Build history of the part. All positions in model axes, mm. Face numbers are marked on the shaded views. Give positions to 0.01 mm unless a question says otherwise; leave off trailing zeros. Order: outer loops, then holes, each group sorted by start corner. A loop starts at its lowest first (then second) coordinate and runs counter-clockwise, first axis right, second up. Notation, with made-up numbers: (-4.5, 31.25) - (38.5, 31.25) arc R28 cw to (38.5, 64.25) - close; hole circle Ø1 at (59.5, 27). An arc over 180 degrees is marked (long way). Answer in a Markdown table with one row per item.
Autodesk Inventor part; units mm, degrees
ref_plane "YZ Plane" through (0, 0, 0) normal (1, 0, 0) x (0, 1, 0)
ref_plane "XZ Plane" through (0, 0, 0) normal (0, 1, 0) x (-1, 0, 0)
ref_plane "XY Plane" through (0, 0, 0) normal (0, 0, 1) x (1, 0, 0)
sketch "Sketch1" plane through (0, 0, 0) normal (0, 0, 1) x (1, 0, 0)
  circle A0 centre (0, 0) radius 15
  dimension "d0" = 30
extrude "Extrusion1" add sketch "Sketch1" along normal blind 40
sketch "Sketch2" plane through (0, 0, 40) normal (0, 0, 1) x (1, 0, 0)
  circle A0 centre (0, 0) radius 4
  dimension "d3" = 8
extrude "Extrusion2" cut sketch "Sketch2" against normal blind 40
sketch "Sketch3" plane through (0, 0, 40) normal (0, 0, 1) x (1, 0, 0)
  circle A0 centre (0, 0) radius 4
  circle A1 centre (0, 0) radius 15
  line L0 (0, 15) -> (1, 15)
  line L1 (0, 15) -> (-1, 15)
  line L2 (-0.0081, 4) -> (0.9843, 3.877)
  line L3 (-0.0081, 4) -> (-1, 3.873)
  line L4 (-1, 3.873) -> (-1, 15)
  line L5 (0.9843, 3.877) -> (1, 15)
  dimension "d8" = 1
  dimension "d9" = 1
  dimension "d10" = 1
  dimension "d11" = 1
extrude "Extrusion3" cut sketch "Sketch3" against normal blind 40 contours L2 A0 | A0 L4 A1 L5 | A0 L3 | A1 L0 L5 | L4 L1 A1 picked at (-0.339, 7.6568)
sketch "Sketch4" plane through (0, 0, 40) normal (0, 0, 1) x (1, 0, 0)
  point P0 (0, 0)
sketch "Sketch5" plane through (1, 14.9666, 0) normal (-1, 0.0014, 0) x (0, 0, 1)
  point P0 (0, -14.968)
sketch "Sketch6" plane through (1, 14.9666, 0) normal (-1, 0.0014, 0) x (0, 0, 1)
  circle A0 centre (36.6199, -3.9195) radius 1.25
  point P0 (0, -14.968)
  dimension "d14" = 2.5
extrude "Extrusion4" cut sketch "Sketch6" against normal blind 15
sketch "Sketch7" plane through (1, 14.9666, 0) normal (-1, 0.0014, 0) x (0, 0, 1)
  circle A0 centre (33.2561, -3.8302) radius 1.25
  point P0 (0, -14.968)
  dimension "d17" = 2.5
extrude "Extrusion5" cut sketch "Sketch7" against normal blind 15
sketch "Sketch8" plane through (1, 14.9666, 0) normal (-1, 0.0014, 0) x (0, 0, 1)
  circle A0 centre (6.8967, -3.6366) radius 1.25
  circle A1 centre (2.3686, -3.6366) radius 1.25
  point P0 (0, -14.968)
  dimension "d20" = 2.5
  dimension "d21" = 2.5
extrude "Extrusion6" cut sketch "Sketch8" against normal blind 30
sketch "Sketch9" plane through (-1, 3.873, 40) normal (1, 0, 0) x (0, 0, -1)
  point P0 (40, -3.873)
sketch "Sketch10" plane through (-1, 3.873, 40) normal (1, 0, 0) x (0, 0, -1)
  ellipse E0 centre (33.1033, 7.4571) end of major axis (31.8533, 7.4571) minor radius 1.25
  circle A0 centre (33.1033, 7.4571) radius 1.25
  ellipse E1 centre (37.6314, 7.4571) end of major axis (36.3814, 7.4571) minor radius 1.25
  circle A1 centre (37.6314, 7.4571) radius 1.25
  ellipse E2 centre (6.7439, 7.2634) end of major axis (5.4939, 7.2634) minor radius 1.25
  circle A2 centre (6.7439, 7.2634) radius 1.25
  ellipse E3 centre (3.3801, 7.1742) end of major axis (2.1301, 7.1742) minor radius 1.25
  circle A3 centre (3.3801, 7.1742) radius 1.25
  point P0 (40, -3.873)
  dimension "d24" = 2.5
  dimension "d25" = 2.5
  dimension "d26" = 2.5
  dimension "d27" = 2.5
extrude "Extrusion7" cut sketch "Sketch10" against normal blind 30
properties part number "Acoplador de servomotor"
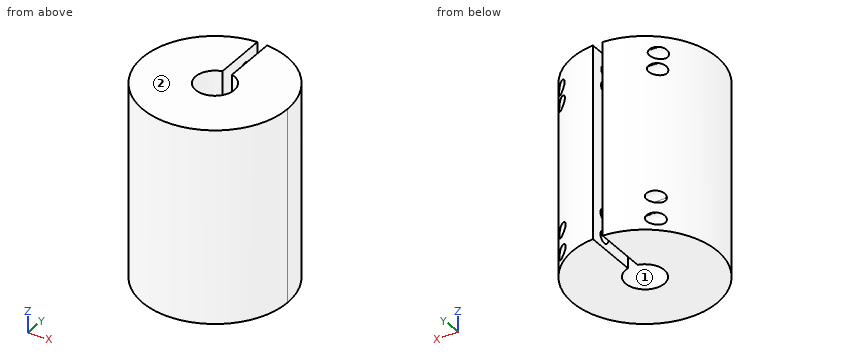
1. Cut at A-A on y = 5.5. Write the cut outline in (x, z), and give its area (3 significant figures).
Check result:
| item | result |
|---|---|
| outline | (-13.96, 0) - (-1, 0) - (-1, 40) - (-13.96, 40) - close; (0.99, 0) - (13.96, 0) - (13.96, 40) - (0.99, 40) - close |
| area | 1,040 mm² |
2. Probe line 1 (Z direction, x = 7.5, y = 10.25); line 2 (X direction, y = 0.25, z = 38.5); line 3 (Y direction, x = 0, z = 22). List the from-to ranges inside material, lowest first.
Check result:
| item | result |
|---|---|
| line 1 | z = 0 to 1.72, 3.01 to 6.25, 7.54 to 32.37, 34.15 to 35.65, 37.59 to 40 |
| line 2 | x = -15 to -3.99, 3.99 to 15 |
| line 3 | y = -15 to -4 |
3. Cut at C-C on z = 13. Write the cut outline in (x, y).
Check result:
| item | result |
|---|---|
| outline | (-1, 3.87) - (-1, 14.97) arc R15 ccw (long way) to (1, 14.97) - (0.98, 3.88) arc R4 cw (long way) to start |
4. Cut at D-D on y = 1.25. Write the cut outline in (x, z).
Check result:
| item | result |
|---|---|
| outline | (-14.95, 0) - (-3.8, 0) - (-3.8, 40) - (-14.95, 40) - close; (3.8, 0) - (14.95, 0) - (14.95, 40) - (3.8, 40) - close |
5. Two-plate mould, pull along Y, no slides. Class the marked faces 1 and 2: +Y half, -Y half, draft (parallel to the pull), parting line (faces both ways), or undercut.
Check result:
| item | result |
|---|---|
| face 1 | undercut |
| face 2 | draft |
6. Cut at B-B on x = 1.5. Count the separate pieces of the cut face and the enclosed holes in it, and give its area (3 significant figures).
Check result:
| item | result |
|---|---|
| separate pieces | 2 |
| enclosed holes | 4 |
| area | 878 mm² |
7. Drop flat-ended pins along their axis: P1, Ø2, axis at x = 6, z = 24, coming from the +Y side; P2, Ø3.5, axis at y = 10.5, z = 10.5, coming from the +X side; P3, Ø6, axis at y = 5, z = 24.5, coming from the -X side; P4, Ø6.5, axis at x = 0, y = 0, coming from the -Z side. Give the stop position or say it passes through.
Check result:
| item | result |
|---|---|
| P1 | stops at y = 14.14 |
| P2 | stops at x = 12.18 |
| P3 | stops at x = -14.87 |
| P4 | passes through |
